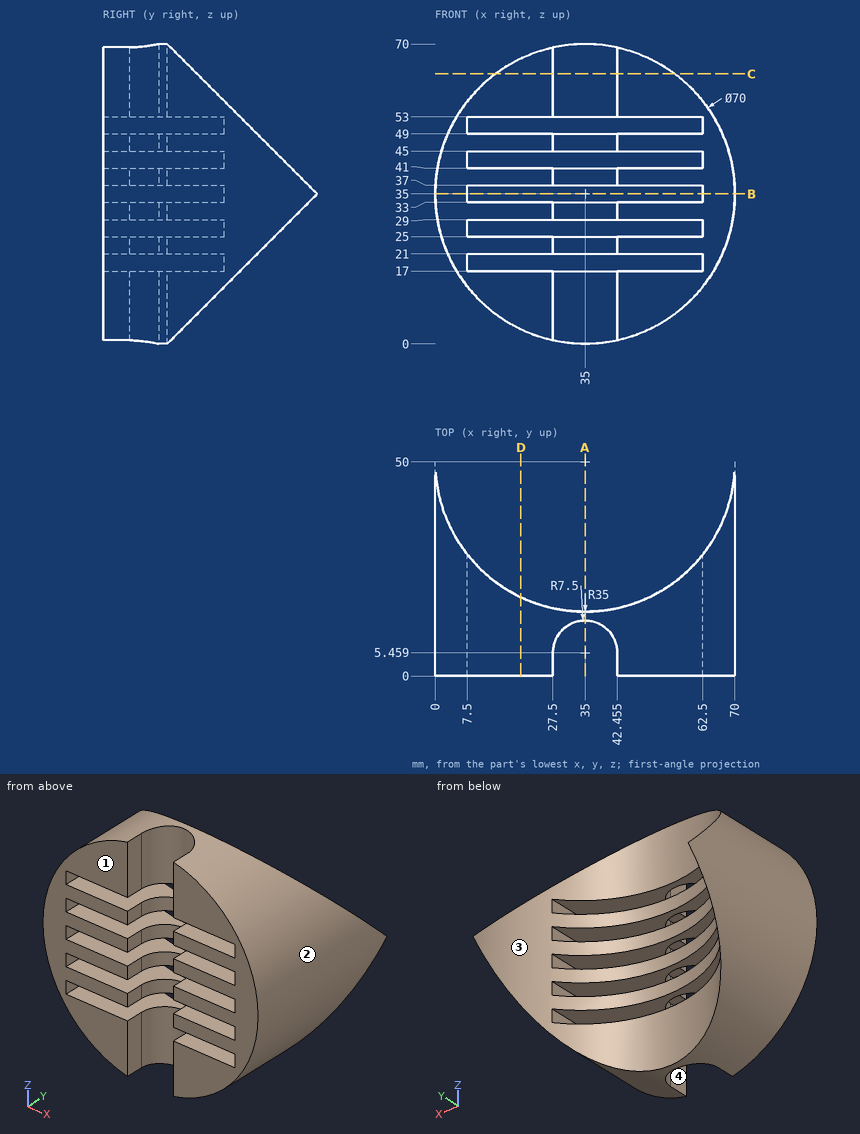
Here's the drawing with two shaded views (mm, measured from the low corner). I have some questions. Give positions to 0.01 mm unless a question says otherwise; leave off trailing zeros. Order: outer loops, then holes, each group sorted by start corner. A loop starts at its lowest first (then second) coordinate and runs counter-clockwise, first axis right, second up. Notation, with made-up numbers: (-36, -25.5) -> (19, -25.5) arc R22 cw to (19, 3.5) -> close; hole circle Ø6 at (-31.5, 58.5). An arc over 180 degrees is marked (long way). Use a Markdown table: item, result. Add a question column.
Item 1: I need wall thicknesses on line 1 (X direction, y = 9.5, z = 36) (1 decimal); line 2 (X direction, y = 43, z = 36) (1 decimal); line 3 (Z direction, x = 49.5, y = 14.5) (1 decimal). Which ranges of each line are inside material? Lowest first, please.
Item 2: Will these pins go through, and if not, where does the flat tip stop? pin 1 (1.5 mm diameter, centred on x = 21.5, z = 14, fed in from +Y); pin 2 (12 mm diameter, centred on y = 11, z = 62, fed in from +X); pin 3 (4 mm diameter, centred on y = 34, z = 30, fed in from +X).
Item 3: Imagine slicing it at B-B on z = 35. Please give me the cut outline in (x, y).
Item 4: Imagine slicing it at A-A on x = 35. Please give me the cut outline in (y, z).
Item 5: If we mould it in two halves opening along X, with no side actions, what happens to the marked faces 1, 2, 3 and 4? For each: pulls with the +X half, pulls with the -X half, needs draft (parallel to the pull), parting line crosses it, or undercut.
Item 6: Imagine slicing it at C-C on z = 63. Please give me the cut outline in (x, y) (1 decimal).
Item 7: Imagine slicing it at D-D on x = 20. Please give me the cut outline in (y, z).
Data:
| question | item | result |
|---|---|---|
| 1 | line 1 | x = 0 to 7.5, 62.5 to 70 |
| 1 | line 2 | x = 0 to 0.7, 69.3 to 70 |
| 1 | line 3 | z = 3.1 to 17, 21 to 25, 29 to 33, 37 to 41, 45 to 49, 53 to 66.9 |
| 2 | pin 1 | stops at y = 18.03 |
| 2 | pin 2 | stops at x = 63 |
| 2 | pin 3 | stops at x = 69.87 |
| 3 | outline | (0, 0) -> (7.5, 0) -> (7.5, 28.35) arc R35 cw to (0, 50) -> close; (62.5, 0) -> (70, 0) -> (70, 50) arc R35 cw to (62.5, 28.35) -> close |
| 4 | outline | (12.96, 0) -> (15, 0) -> (15, 17) -> (12.96, 17) -> close; (12.96, 21) -> (15, 21) -> (15, 25) -> (12.96, 25) -> close; (12.96, 29) -> (15, 29) -> (15, 33) -> (12.96, 33) -> close; (12.96, 37) -> (15, 37) -> (15, 41) -> (12.96, 41) -> close; (12.96, 45) -> (15, 45) -> (15, 49) -> (12.96, 49) -> close; (12.96, 53) -> (15, 53) -> (15, 70) -> (12.96, 70) -> close |
| 5 | face 1 | needs draft |
| 5 | face 2 | parting line crosses it |
| 5 | face 3 | undercut |
| 5 | face 4 | undercut |
| 6 | outline | (14, 0) -> (27.5, 0) -> (27.5, 5.5) arc R7.5 cw to (42.5, 6.3) -> (42.5, 0) -> (56, 0) -> (56, 22) arc R35 cw to (14, 22) -> close |
| 7 | outline | (0, 3.38) -> (18.38, 3.38) -> (18.38, 17) -> (0, 17) -> close; (0, 21) -> (18.38, 21) -> (18.38, 25) -> (0, 25) -> close; (0, 29) -> (18.38, 29) -> (18.38, 33) -> (0, 33) -> close; (0, 37) -> (18.38, 37) -> (18.38, 41) -> (0, 41) -> close; (0, 45) -> (18.38, 45) -> (18.38, 49) -> (0, 49) -> close; (0, 53) -> (18.38, 53) -> (18.38, 66.62) -> (0, 66.62) -> close |
